Drawing for the job (mm, zero at the part's lowest x, y, z). A direction names the side the tool comes from. Round coordinates to 2 decimals unless told otherwise and drop trailing zeros. Order: outer loops, then holes, each group sorted by start corner. A loop starts at its lowest first (then second) coordinate and runs counter-clockwise, first axis right, second up. Notation, with made-up numbers: M 26.5,26 L 67.5,26 A19 ccw 67.5,58 Z; hole C 47,-11 d9. An arc over 180 degrees is marked long. One line per item, written item: value. Start each with the question number.
Item 1: Tool access for the marked faces 4 and 5: list every direction of +Z, -Z, +X, -X, +Y, -Y with a clear straight run to the whole face (end or side of a thin tool).
Item 2: Band-saw the part on B-B, the plane z = 16. Write the cut outline in (x, y).
Item 3: Band-saw the part on D-D, the plane y = 18. Write the cut outline in (x, z), then the cut area to 3 significant figures.
Item 4: Pin check, flat tips, straight feed: pin 1 (4 mm diameter, centred on x = 43.5, y = 46.5, fed in from -Z); pin 2 (4 mm diameter, centred on y = 32.5, z = 9.5, fed in from -X); pin 3 (10 mm diameter, centred on y = 30, z = 16.5, fed in from +X); pin 4 (1.9 mm diameter, centred on x = 70, y = 60, fed in from -Z). Stop position of each tip, or through.
Item 5: Band-saw the part on A-A, the plane x = 97.5. Write the cut outline in (y, z), then the cut area to 3 significant figures.
Item 6: Probe L1, parallel to Z at x = 121, y = 74; L2, parallel to Y at x = 59, z = 11; L3, parallel to Y at x = 70, z = 31. List the from-to ranges inside material, lowest first.
Item 7: Two-plate mould, pull along Y, no slides. Class the marked faces 1, 2 and 3: +Y half, -Y half, draft (parallel to the pull), parting line (faces both ways), or undercut.
Item 8: Band-saw the part on C-C, the plane x = 80. Write the cut outline in (y, z), then the cut area to 3 significant figures.
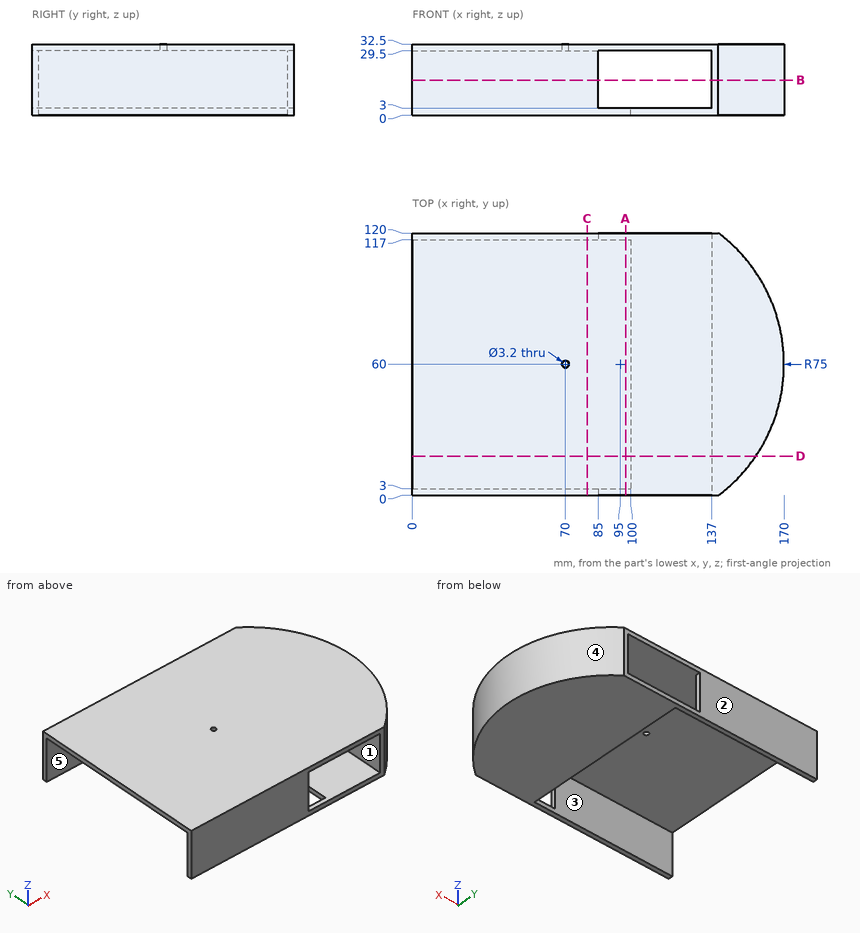
Output:
1. face 4: +Z, -Z, +X
1. face 5: -Z, -X
2. outline: M 0,0 L 85,0 L 85,3 L 0,3 Z; M 0,117 L 85,117 L 85,120 L 0,120 Z; M 137,0 L 140,0 A75 ccw 140,120 L 137,120 Z
3. outline: M 0,29.5 L 137,29.5 L 137,3 L 100,3 L 100,0 L 157.14,0 L 157.14,32.5 L 0,32.5 Z
3. area: 1,180 mm²
4. pin 1: stops at z = 29.5
4. pin 2: stops at x = 137
4. pin 3: stops at x = 165.71
4. pin 4: passes through
5. outline: M 0,0 L 3,0 L 3,3 L 0,3 Z; M 0,29.5 L 120,29.5 L 120,32.5 L 0,32.5 Z; M 117,0 L 120,0 L 120,3 L 117,3 Z
5. area: 378 mm²
6. L1: z = 0 to 3, 29.5 to 32.5
6. L2: y = 0 to 3, 117 to 120
6. L3: y = 0 to 58.4, 61.6 to 120
7. face 1: draft
7. face 2: +Y half
7. face 3: undercut
8. outline: M 0,0 L 3,0 L 3,29.5 L 117,29.5 L 117,0 L 120,0 L 120,32.5 L 0,32.5 Z
8. area: 537 mm²
